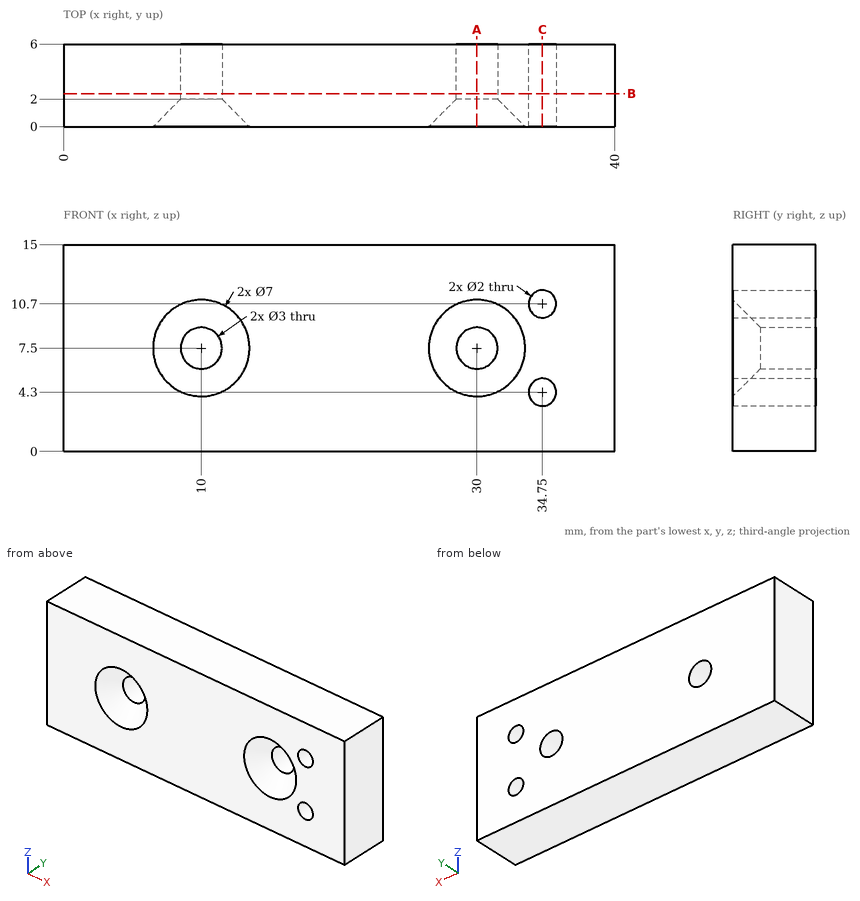
Part print with two shaded views. Sizes in mm from the minimum x, y, z corner. Round coordinates to 2 decimals unless told otherwise and drop trailing zeros. Loops run counter-clockwise (first coordinate to the right, second up) from the corner with the lowest first, then second, coordinate; pieces in that order, holes last.
Item 1: Saw through at B-B (y = 2.4). List the corners of the cut face in (x, z), then the cut area to 3 significant figures.
Item 2: Saw through at A-A (x = 30). List the corners of the cut face in (y, z).
Item 3: Pin check, flat tip, straight feed: P1, Ø5, axis at x = 30, z = 7.5, coming from the -Y side. Stop position of the tip, or through.
Item 4: Drill centre lines: line 1 along Z through (x, y) = (34.75, 1.45); line 2 along Z through (x, y) = (35.5, 5.75); line 3 along X through (y, z) = (4.95, 6.75). Where is each one in solid material? Low to high.
Item 5: Saw through at C-C (x = 34.75). List the corners of the cut face in (y, z).
Worked answers:
1. outline: (0, 0) - (40, 0) - (40, 15) - (0, 15) - close; hole circle Ø3 at (10, 7.5); hole circle Ø3 at (30, 7.5); hole circle Ø2 at (34.75, 4.3); hole circle Ø2 at (34.75, 10.7)
1. area: 580 mm2
2. outline: (0, 0) - (6, 0) - (6, 6) - (2, 6) - (0, 4) - close; (0, 11) - (2, 9) - (6, 9) - (6, 15) - (0, 15) - close
3. P1: stops at y = 1
4. line 1: z = 0 to 3.3, 5.3 to 9.7, 11.7 to 15
4. line 2: z = 0 to 3.64, 4.96 to 10.04, 11.36 to 15
4. line 3: x = 0 to 8.7, 11.3 to 28.7, 31.3 to 40
5. outline: (0, 0) - (6, 0) - (6, 3.3) - (0, 3.3) - close; (0, 5.3) - (6, 5.3) - (6, 9.7) - (0, 9.7) - close; (0, 11.7) - (6, 11.7) - (6, 15) - (0, 15) - close
